The model under review builds one solid part; all positions refer to its coordinate system, in mm. Round coordinates to 2 decimals unless told otherwise and drop trailing zeros. Order: outer loops, then holes, each group sorted by start corner. A loop starts at its lowest first (then second) coordinate and runs counter-clockwise, first axis right, second up. Notation, with made-up numbers: M 6.25,-13 L 13.25,-13 A27 cw 13.25,6 Z; hole C 1,-8.5 d4. An arc over 180 degrees is marked long. One line per item, written item: value. Start each with the question number.
from build123d import *

# Parameters (mm, degrees)
SKETCH1_W           = 66.34988
SKETCH1_H           = 38.1
BOSS_EXTRUDE1_DEPTH = 3.175


with BuildPart() as part:
    # Sketch1 → Boss-Extrude1 (new body)
    with BuildSketch(Plane.XY):
        Rectangle(SKETCH1_W, SKETCH1_H)
        Polygon((11.43, -15.875), (22.225000466, -9.642503575), (22.225000466, 2.822489275), (11.43, 9.0549857), (0.634999534, 2.822489275), (0.634999534, -9.642503575), align=None, mode=Mode.SUBTRACT)
        Polygon((-0.634999534, -9.642503575), (-11.43, -15.875), (-22.225000466, -9.642503575), (-22.225000466, 2.822489275), (-11.43, 9.0549857), (-0.634999534, 2.822489275), align=None, mode=Mode.SUBTRACT)
    extrude(amount=BOSS_EXTRUDE1_DEPTH)


solid = part.part
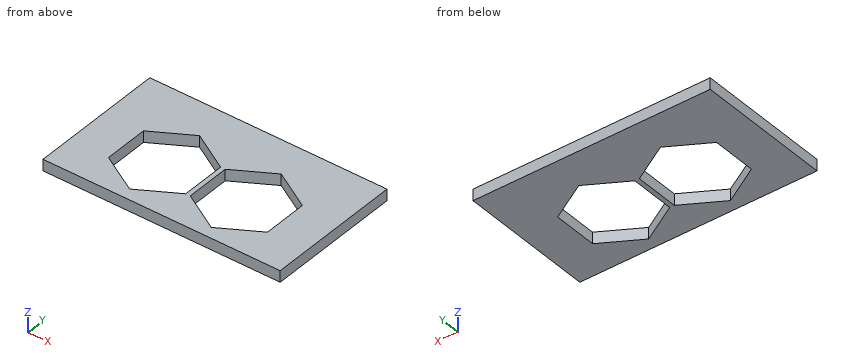
Item 1: Clearance check with flat-ended pins moving along their axes: P1, Ø1, axis at x = -15, y = -11, coming from the -Z side; P2, Ø1, axis at x = -5, y = 12.5, coming from the -Z side. State where each tip first meets the part, or that it passes through.
Item 2: Consider section C-C, the plane z = 2.4. Count the separate pieces of the cut face and the enclosed holes in it, then the cut area to 3 significant figures.
Item 3: Wall thickness on L1, parallel to X at y = -3, z = 2.2 (3 decimals); L2, parallel to X at y = 4, z = 0.9; L3, parallel to Y at x = -8.5, z = 1.35: over which ranges is each line inside the solid? List them lowest first.
Item 4: Consider section B-B, the plane y = -1.5. Give the boundary of the cut face in (x, z) (3 decimals).
Item 5: Consider section D-D, the plane x = 21.5. Give the boundary of the cut face in (y, z) (3 decimals).
Item 6: Consider section A-A, the plane x = -14.5. Give the boundary of the cut face in (y, z) (3 decimals).
Computed:
1. P1: passes through
1. P2: stops at z = 0
2. separate pieces: 1
2. enclosed holes: 2
2. area: 1,720 mm^2
3. L1: x = -33.175 to -22.225, -0.635 to 0.635, 22.225 to 33.175
3. L2: x = -33.17 to -20.19, -2.67 to 2.67, 20.19 to 33.17
3. L3: y = -19.05 to -14.18, 7.36 to 19.05
4. outline: M -33.175,0 L -22.225,0 L -22.225,3.175 L -33.175,3.175 Z; M -0.635,0 L 0.635,0 L 0.635,3.175 L -0.635,3.175 Z; M 22.225,0 L 33.175,0 L 33.175,3.175 L 22.225,3.175 Z
5. outline: M -19.05,0 L -10.061,0 L -10.061,3.175 L -19.05,3.175 Z; M 3.241,0 L 19.05,0 L 19.05,3.175 L 3.241,3.175 Z
6. outline: M -19.05,0 L -14.103,0 L -14.103,3.175 L -19.05,3.175 Z; M 7.283,0 L 19.05,0 L 19.05,3.175 L 7.283,3.175 Z
